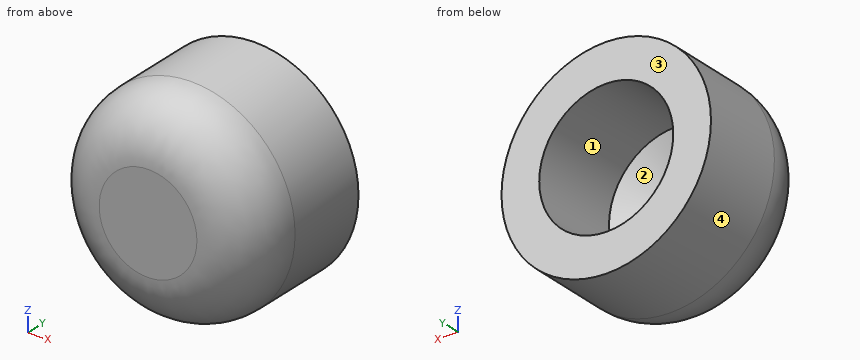
```python
from build123d import *

# Parameters (mm, degrees)
F0_R     = 9.525
F0_R_2   = 6.096
F1_DEPTH = 12.7
F2_R     = 5.08
F3_D     = 12.192
F3_DEPTH = 8.382
F3_TIP   = 3.6628463336


with BuildPart() as f1:
    # F0 (on Front) → F1 (new body)
    with BuildSketch(Plane.XZ):
        Circle(F0_R)
        Circle(F0_R_2, mode=Mode.SUBTRACT)
        Circle(F0_R_2)
    extrude(amount=F1_DEPTH)

    # F2
    f2_edges = [f1.edges().sort_by_distance(p)[0] for p in [
        (-9.525, -12.7, 0),
    ]]
    fillet(f2_edges, radius=F2_R)

    # F3
    with Locations(Plane(origin=(0, 0, 0), x_dir=(1, 0, 0), z_dir=(0, 1, 0))):
        with Locations((0, 0)):
            Hole(F3_D / 2, depth=F3_DEPTH)
            with Locations((0, 0, -(F3_DEPTH + F3_TIP / 2))):  # 118° drill point
                Cone(0, F3_D / 2, F3_TIP, mode=Mode.SUBTRACT)


solid = f1.part
```
Check sheet for the modelled part. Datum: model origin and axes. Units: mm. Face numbers are marked on the shaded views. Coordinates: 2 decimals unless noted, no trailing zeros. Order: outer loops, then holes, each group sorted by start corner. A loop starts at its lowest first (then second) coordinate and runs counter-clockwise, first axis right, second up. Notation, with made-up numbers: (-3, -19) -> (15, -19) arc R23 cw to (15, 9) -> close; hole circle Ø7 at (58.5, 82.5). An arc over 180 degrees is marked (long way). Write item = value, one per line. Start each with the question number.
1) Mould release check, pull along X, two halves, no side actions. Record for the marked faces 1, 2, 3 and 4: +X half, -X half, draft (parallel to the pull), parting line (faces both ways), or undercut.
2) Cross-section at A-A (y = -3.5). Enter the section's corners in (x, z) (3 decimals).
3) Go/stop test with flat-tipped pins: P1, Ø4, axis at x = 6.5, y = -6, coming from the -Z side (3 decimals); P2, Ø3, axis at y = -2.5, z = 4.5, coming from the +X side; P3, Ø2, axis at x = 7, y = -2, coming from the +Z side; P4, Ø10, axis at x = -3.5, z = 6, coming from the -Y side. Record where each tip stops, or that it passes through.
4) Material ranges on L1, parallel to Z at x = 0, y = -4 (3 decimals); L2, parallel to X at y = -11.25, z = -0.5; L3, parallel to X at y = -1.5, z = 1.75, recorded low to high.
Ans:
q1.face_1 = undercut
q1.face_2 = undercut
q1.face_3 = draft
q1.face_4 = parting line
q2.outline = circle Ø19.05 at (0, 0); hole circle Ø12.192 at (0, 0)
q3.P1 = -8.395
q3.P2 = 9.04
q3.P3 = 7.4
q3.P4 = -12.7
q4.L1 = -9.525 to -6.096, 6.096 to 9.525
q4.L2 = -7.98 to -1.22, 1.22 to 7.98
q4.L3 = -9.36 to -5.84, 5.84 to 9.36
